```python
from build123d import *

# Parameters (mm, degrees)
SKETCH_1_W                   = 140
SKETCH_1_H                   = 120
EXTRUDE_1_DEPTH              = 10
HOLE_WIZARD_M6_1_D           = 6.6
HOLE_WIZARD_M6_1_CSINK_D     = 18.6
HOLE_WIZARD_M6_1_CSINK_ANGLE = 90
SKETCH_4_W                   = 5
SKETCH_4_H                   = 40
EXTRUDE_2_DEPTH              = 8
HOLE_WIZARD_M3_2_D           = 3.4
HOLE_WIZARD_M3_2_DEPTH       = 5
SKETCH_13_R                  = 5
CUT_EXTRUDE_5_DEPTH          = 3
HOLE_WIZARD_M4_1_D           = 4.5
HOLE_WIZARD_M4_1_CBORE_D     = 9
HOLE_WIZARD_M4_1_CBORE_DEPTH = 3.1
SKETCH_21_W                  = 5
SKETCH_21_H                  = 40
EXTRUDE_4_DEPTH              = 8
HOLE_WIZARD_M3_4_D           = 3.4
SKETCH_24_W                  = 3.5
SKETCH_24_H                  = 20
SKETCH_24_W_2                = 4
SKETCH_24_H_2                = 24
CUT_EXTRUDE_6_DEPTH          = 81
CUT_EXTRUDE_6_DEPTH_BACK     = 61
FILLET_1_R                   = 10
FILLET_2_R                   = 2


with BuildPart() as part:
    # 스케치1 → 보스-돌출1 (new body)
    with BuildSketch(Plane.XY):
        Rectangle(SKETCH_1_W, SKETCH_1_H)
    extrude(amount=EXTRUDE_1_DEPTH)

    # M6 접시 머리 나사용 카운터싱크1 (through all)
    with Locations(Plane.XY.offset(10)):
        with Locations((0, 25), (25, 0), (0, -25), (-25, 0)):
            CounterSinkHole(HOLE_WIZARD_M6_1_D / 2, HOLE_WIZARD_M6_1_CSINK_D / 2, counter_sink_angle=HOLE_WIZARD_M6_1_CSINK_ANGLE)

    # 스케치4 → 보스-돌출2 (add)
    with BuildSketch(Plane.XY.offset(10)):
        with Locations((-12.5, -35)):
            Rectangle(SKETCH_4_W, SKETCH_4_H)
    extrude(amount=EXTRUDE_2_DEPTH)

    # M3 여유 구멍2
    with Locations(Plane(origin=(-10, 0, 0), x_dir=(0, 0, -1), z_dir=(1, 0, 0))):
        with Locations((-15.5, -51), (-15.5, -20)):
            Hole(HOLE_WIZARD_M3_2_D / 2, depth=HOLE_WIZARD_M3_2_DEPTH)

    # 스케치13 → 컷-돌출5 (cut)
    with BuildSketch(Plane.XY.offset(10)):
        with Locations((-60, 50)):
            Circle(SKETCH_13_R)
        with Locations((60, 50)):
            Circle(SKETCH_13_R)
        with Locations((60, -50)):
            Circle(SKETCH_13_R)
        with Locations((-60, -50)):
            Circle(SKETCH_13_R)
    extrude(amount=-CUT_EXTRUDE_5_DEPTH, mode=Mode.SUBTRACT)

    # M4 남비 머리 나사용 카운터보어1 (through all)
    with Locations(Plane(origin=(0, 0, 0), x_dir=(-1, 0, 0), z_dir=(0, 0, -1))):
        with Locations((-60, 50), (60, 50), (60, -50), (-60, -50)):
            CounterBoreHole(HOLE_WIZARD_M4_1_D / 2, HOLE_WIZARD_M4_1_CBORE_D / 2, HOLE_WIZARD_M4_1_CBORE_DEPTH)

    # 스케치21 → 보스-돌출4 (add)
    with BuildSketch(Plane.XY.offset(10)):
        with Locations((12, 35)):
            Rectangle(SKETCH_21_W, SKETCH_21_H)
    extrude(amount=EXTRUDE_4_DEPTH)

    # M3 여유 구멍4 (through all)
    with Locations(Plane.ZY.offset(-9.5)):
        with Locations((15.5, 50), (15.5, 19)):
            Hole(HOLE_WIZARD_M3_4_D / 2)

    # 스케치24 → 컷-돌출6 (cut, two sides)
    with BuildSketch(Plane(origin=(-10, 0, 0), x_dir=(0, 0, -1), z_dir=(1, 0, 0))) as cut_extrude_6_sk:
        with Locations((-16.25, -35)):
            Rectangle(SKETCH_24_W, SKETCH_24_H)
        with Locations((-16, 35)):
            Rectangle(SKETCH_24_W_2, SKETCH_24_H_2)
    extrude(amount=CUT_EXTRUDE_6_DEPTH, mode=Mode.SUBTRACT)
    extrude(cut_extrude_6_sk.sketch, amount=-CUT_EXTRUDE_6_DEPTH_BACK, mode=Mode.SUBTRACT)

    # 필렛1
    fillet_1_edges = [part.edges().sort_by_distance(p)[0] for p in [
        (70, -60, 5),
        (-70, -60, 5),
        (-70, 60, 5),
        (70, 60, 5),
    ]]
    fillet(fillet_1_edges, radius=FILLET_1_R)

    # 필렛2
    fillet_2_edges = [part.edges().sort_by_distance(p)[0] for p in [
        (12, 47, 18),
        (12, 23, 18),
        (-12.5, -25, 18),
        (-12.5, -45, 18),
    ]]
    fillet(fillet_2_edges, radius=FILLET_2_R)


solid = part.part
```
Verification items for the finished model (mm, model axes). A direction names the side the tool comes from. Coordinates: 2 decimals unless noted, no trailing zeros. Write each loop counter-clockwise with the first axis right and the second up, starting at its lowest first coordinate (ties: lowest second). Pieces come first, ordered by that corner, then holes. Notation, with made-up numbers: M 66.5,89 L 119.5,89 A16 ccw 119.5,108 Z; hole C 63,40.25 d4. An arc over 180 degrees is marked long. Answer as a JSON object with one key per item and string values. Group by question number.
(1) Material ranges on line 1 (Y direction, x = -60, z = 7.75); line 2 (Y direction, x = 0, z = 2.3); line 3 (Y direction, x = 14, z = 15.5), recorded low to high.
(2) Cross-section at B-B, the plane y = 25. Record the cut outline in (x, z).
(3) Cross-section at A-A, the plane x = -25. Record the cut outline in (y, z).
(4) Tool access check on faces 5 (the face through (-15, -35, 13)), 6 (the face through (14.5, 35, 13)), 7 (the face through (12, 55, 14)), 8 (the face through (-60.651, 54.957, 8.521)), 9 (the face through (57.92, -53.99, 1.53)). Record the directions out of +Z, -Z, +X, -X, +Y, -Y that give a thin tool (end or side, any length) a straight path to the whole face; none if there is none.
(5) Gauge pin test, flat ends, axial feed: pin 1 (4 mm diameter, centred on y = 36, z = 14.5, fed in from -X); pin 2 (10.5 mm diameter, centred on x = 25, y = 0, fed in from -Z); pin 3 (1.6 mm diameter, centred on x = 11, z = 15, fed in from +Y); pin 4 (2.5 mm diameter, centred on y = 43.5, z = 14, fed in from +X). Record the tip position at first contact, or that the pin passes through.
(6) Release check for a two-part mould opening along Y. For faces 1 (the face through (12, 35, 14)), 2 (the face through (66.99, -57.15, 5.07)), 3 (the face through (59.71, -47.77, 5.08)), 4 (the face through (-10, -35, 13)) record: +Y half, -Y half, draft (parallel to the pull), parting line (faces both ways), or undercut.
Reply:
{
 "1": {"line 1": "-60 to -55, -45 to 45, 55 to 60", "line 2": "-60 to -28.3, -21.7 to 21.7, 28.3 to 60", "line 3": "15 to 17.3, 20.7 to 23, 47 to 48.3, 51.7 to 55"},
 "2": {"outline": "M -70,0 L -3.3,0 L -3.3,4 L -9.3,10 L -70,10 Z; M 3.3,0 L 70,0 L 70,10 L 14.5,10 L 14.5,14 L 9.5,14 L 9.5,10 L 9.3,10 L 3.3,4 Z"},
 "3": {"outline": "M -60,0 L -3.3,0 L -3.3,4 L -9.3,10 L -60,10 Z; M 3.3,0 L 60,0 L 60,10 L 9.3,10 L 3.3,4 Z"},
 "4": {"face 5": "+Z, -X, +Y, -Y", "face 6": "+Z, +X, +Y, -Y", "face 7": "+Z, +X, -X, +Y", "face 8": "+Z", "face 9": "-Z"},
 "5": {"pin 1": "x = 9.5", "pin 2": "z = 0", "pin 3": "y = 55", "pin 4": "x = 14.5"},
 "6": {"face 1": "undercut", "face 2": "-Y half", "face 3": "undercut", "face 4": "draft"}
}
